Answer from the drawing. Dimensions are ordinates in mm from the lowest x, y and z of the part. Round coordinates to 2 decimals unless told otherwise and drop trailing zeros. Write each loop counter-clockwise with the first axis right and the second up, starting at its lowest first coordinate (ties: lowest second). Pieces come first, ordered by that corner, then holes. Notation, with made-up numbers: (4.5, -37) - (25.5, -37) arc R15 cw to (25.5, -22) - close; hole circle Ø1 at (13, 74.25). An arc over 180 degrees is marked (long way). Return JSON: item names as keys, results as strings. Group by question number.
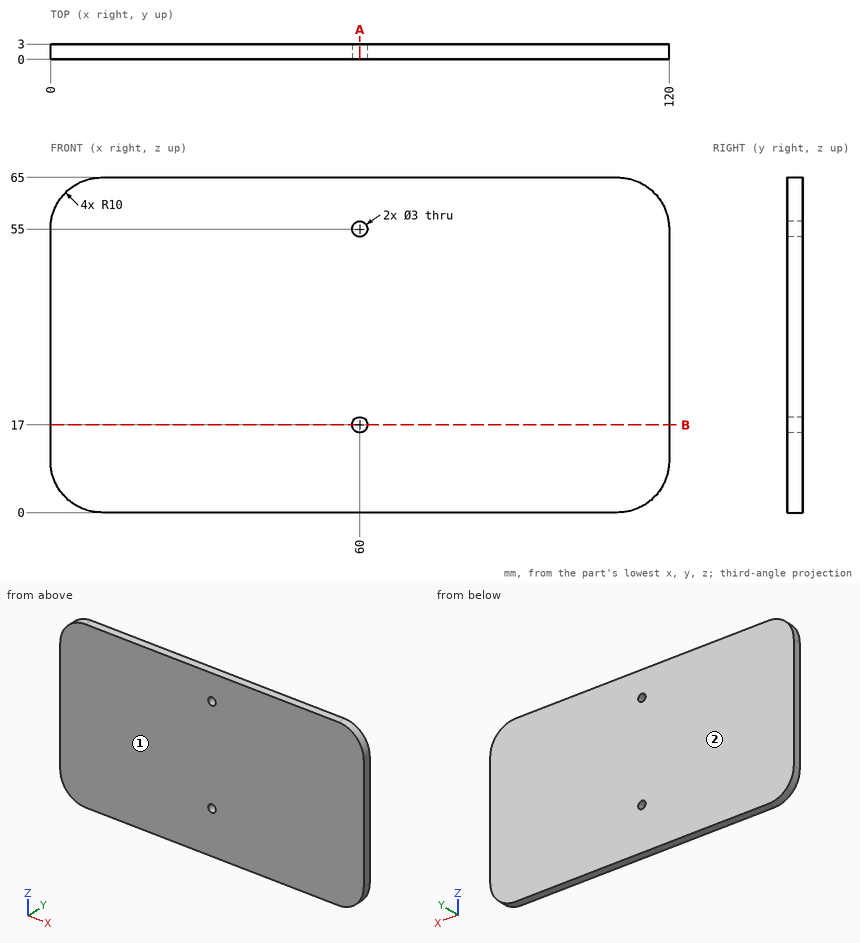
(1) Find section B-B (z = 17). Write down the section's boundary in (x, y), plus the area to 3 significant figures.
(2) Consider line 1 (Z direction, x = 60, y = 1); line 2 (X direction, y = 1.5, z = 17); line 3 (X direction, y = 1.95, z = 18). Determine where each line is inside the solid, lowest interval first.
(3) Find section A-A (x = 60). Write down the section's boundary in (y, z).
(4) Flat-ended cylindrical pins translate along their axes: pin 1 (1.8 mm diameter, centred on x = 60, z = 17, fed in from +Y); pin 2 (1.5 mm diameter, centred on y = 0.5, z = 57.5, fed in from -X). Find the tip coordinate at first contact, or state that the pin passes through.
(5) Determine the mould class of the marked faces 1 and 2 for opening direction Y: +Y half, -Y half, draft (parallel to the pull), parting line (faces both ways), or undercut.
Check sheet entries:
{
 "1": {"outline": "(0, 0) - (58.5, 0) - (58.5, 3) - (0, 3) - close; (61.5, 0) - (120, 0) - (120, 3) - (61.5, 3) - close", "area": "351 mm^2"},
 "2": {"line 1": "z = 0 to 15.5, 18.5 to 53.5, 56.5 to 65", "line 2": "x = 0 to 58.5, 61.5 to 120", "line 3": "x = 0 to 58.88, 61.12 to 120"},
 "3": {"outline": "(0, 0) - (3, 0) - (3, 15.5) - (0, 15.5) - close; (0, 18.5) - (3, 18.5) - (3, 53.5) - (0, 53.5) - close; (0, 56.5) - (3, 56.5) - (3, 65) - (0, 65) - close"},
 "4": {"pin 1": "passes through", "pin 2": "stops at x = 0.15"},
 "5": {"face 1": "-Y half", "face 2": "+Y half"}
}
